Here's the drawing with two shaded views (mm, measured from the low corner). I have some questions. Coordinates: 2 decimals unless noted, no trailing zeros. Loops run counter-clockwise (first coordinate to the right, second up) from the corner with the lowest first, then second, coordinate; pieces in that order, holes last.
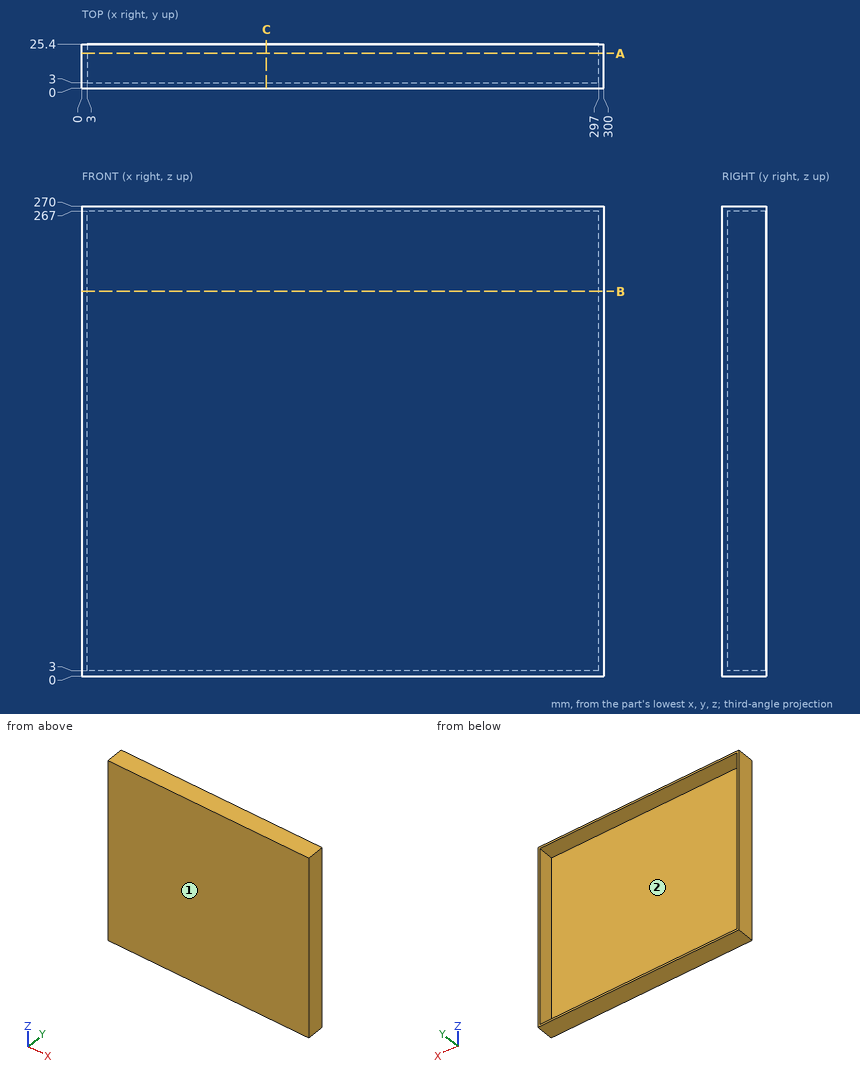
Q1. Suppose I cut it at A-A on y = 20. Write out the boundary of the cut face in (x, z).
Q2. Please list where these lines run through material, in increasing order: probe 1 along X at (y, z) = (18.5, 99); probe 2 along Z at (x, y) = (218, 15.25); probe 3 along Y at (x, z) = (112, 34).
Q3. Will this pin go through, and if not, where does the flat tip stop? P1, Ø1, axis at x = 189, z = 43.5, coming from the +Y side.
Q4. Suppose I cut it at B-B on z = 221. Write out the boundary of the cut face in (x, y), and give its area (3 significant figures).
Q5. Suppose I cut it at C-C on x = 106. Write out the boundary of the cut face in (y, z).
Q6. We'd pull the mould along X, two halves only. Please class the marked faces 1 and 2: pulls with the +X half, pulls with the -X half, needs draft (parallel to the pull), parting line crosses it, or undercut.
Check values:
1. outline: (0, 0) - (300, 0) - (300, 270) - (0, 270) - close; hole (3, 3) - (297, 3) - (297, 267) - (3, 267) - close
2. probe 1: x = 0 to 3, 297 to 300
2. probe 2: z = 0 to 3, 267 to 270
2. probe 3: y = 0 to 3
3. P1: stops at y = 3
4. outline: (0, 0) - (300, 0) - (300, 25.4) - (297, 25.4) - (297, 3) - (3, 3) - (3, 25.4) - (0, 25.4) - close
4. area: 1,030 mm2
5. outline: (0, 0) - (25.4, 0) - (25.4, 3) - (3, 3) - (3, 267) - (25.4, 267) - (25.4, 270) - (0, 270) - close
6. face 1: needs draft
6. face 2: undercut
